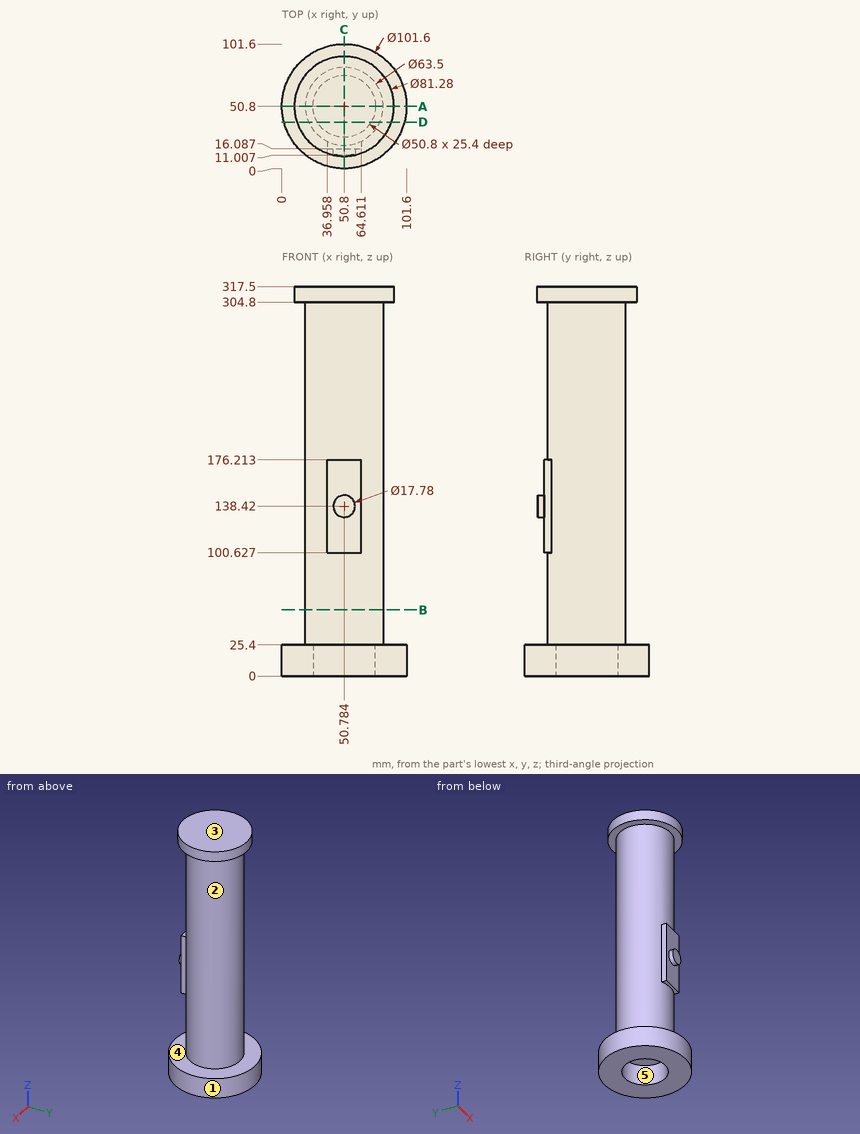
Study the drawing (mm; zero at the part's minimum x, y, z) and answer. A direction names the side the tool comes from. Coordinates: 2 decimals unless noted, no trailing zeros. Write each loop counter-clockwise with the first axis right and the second up, starting at its lowest first coordinate (ties: lowest second). Pieces come first, ordered by that corner, then holes. Notation, with made-up numbers: (43, -36) - (73, -36) arc R30 ccw to (73, -8) - close; hole circle Ø4 at (44, 53.25). An arc over 180 degrees is marked (long way). Answer as a JSON object with one key per item and string values. Group by question number.
1. Which of the six approach directions +Z, -Z, +X, -X, +Y, -Y give full straight-line access (tool end or side, diameter ignored) to the marked faces 1 and 2?
2. A cutting plane is placed at D-D (y = 38). Determine the outline of the cut face in (x, z) (1 decimal).
3. A cutting plane is placed at C-C (x = 50.8). Determine the outline of the cut face in (y, z), plus the area to 3 significant figures.
4. A cutting plane is placed at A-A (y = 50.8). Determine the outline of the cut face in (x, z).
5. The mould has two halves that part along Z. Classify the marked faces 3, 4 and 5: +Z half, -Z half, draft (parallel to the pull), parting line (faces both ways), or undercut.
6. Each of these flat-tipped pins is pushed along its axis until it touches: P1, Ø19.5, axis at x = 53.5, z = 142.5, coming from the -Y side; P2, Ø2, axis at y = 74, z = 201.5, coming from the -X side; P3, Ø1.8, axis at y = 18, z = 150, coming from the +X side. Where does it stop, or does it pass through?
7. Consider L1, parallel to Z at x = 23, y = 75; L2, parallel to X at y = 50, z = 12; L3, parallel to Y at x = 50.8, z = 5.75. Determine where each line is inside the solid, lowest interval first. Write a range as [from, to].
8. A cutting plane is placed at B-B (z = 54). Determine the outline of the cut face in (x, y), plus the area to 3 significant figures.
Worked out:
{
 "1": {"face 1": "+Z, -Z", "face 2": "none"},
 "2": {"outline": "(1.6, 0) - (28.9, 0) - (28.9, 25.4) - (72.7, 25.4) - (72.7, 0) - (100, 0) - (100, 25.4) - (79.9, 25.4) - (79.9, 304.8) - (89.4, 304.8) - (89.4, 317.5) - (12.2, 317.5) - (12.2, 304.8) - (21.7, 304.8) - (21.7, 25.4) - (1.6, 25.4) - close"},
 "3": {"outline": "(0, 0) - (25.4, 0) - (25.4, 25.4) - (76.2, 25.4) - (76.2, 0) - (101.6, 0) - (101.6, 25.4) - (82.55, 25.4) - (82.55, 304.8) - (91.44, 304.8) - (91.44, 317.5) - (10.16, 317.5) - (10.16, 304.8) - (19.05, 304.8) - (19.05, 176.21) - (16.09, 176.21) - (16.09, 147.31) - (11.01, 147.31) - (11.01, 129.53) - (16.09, 129.53) - (16.09, 100.63) - (19.05, 100.63) - (19.05, 25.4) - (0, 25.4) - close", "area": "20,400 mm²"},
 "4": {"outline": "(0, 0) - (25.4, 0) - (25.4, 25.4) - (76.2, 25.4) - (76.2, 0) - (101.6, 0) - (101.6, 25.4) - (82.55, 25.4) - (82.55, 304.8) - (91.44, 304.8) - (91.44, 317.5) - (10.16, 317.5) - (10.16, 304.8) - (19.05, 304.8) - (19.05, 25.4) - (0, 25.4) - close"},
 "5": {"face 3": "+Z half", "face 4": "undercut", "face 5": "draft"},
 "6": {"P1": "stops at y = 11.01", "P2": "stops at x = 28.1", "P3": "stops at x = 64.61"},
 "7": {"L1": "z = [0, 25.4], [304.8, 317.5]", "L2": "x = [0.01, 25.41], [76.19, 101.59]", "L3": "y = [0, 25.4], [76.2, 101.6]"},
 "8": {"outline": "circle Ø63.5 at (50.8, 50.8)", "area": "3,170 mm²"}
}
